Build history of the part. All positions in model axes, mm. Face numbers are marked on the shaded views. A direction names the side the tool comes from. Give positions to 0.01 mm unless a question says otherwise; leave off trailing zeros. Loops run counter-clockwise (first coordinate to the right, second up) from the corner with the lowest first, then second, coordinate; pieces in that order, holes last. Notation, with made-up numbers: (51, 8.5) -> (109, 8.5) arc R13 ccw to (109, 13.5) -> close; hole circle Ø6 at (51, 63.5). An arc over 180 degrees is marked (long way). Answer in a Markdown table with one row per item. Add a question column.
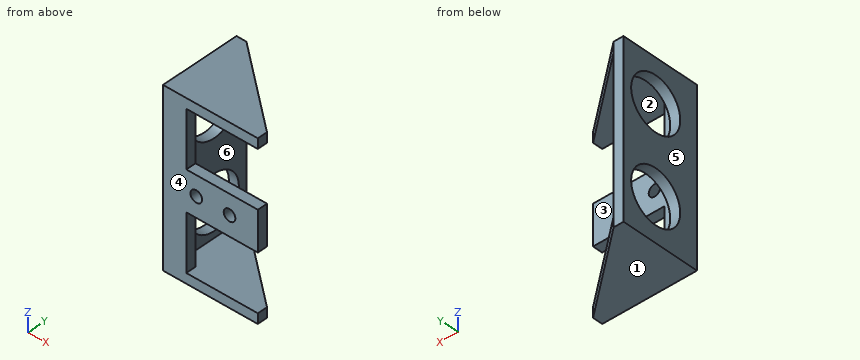
from build123d import *

# Parameters (mm, degrees)
CROQUIS1_W              = 52
CROQUIS1_H              = 21
CROQUIS1_R              = 8.025
SALIENTE_EXTRUIR1_DEPTH = 3
CROQUIS2_W              = 3
CROQUIS2_H              = 21
SALIENTE_EXTRUIR2_DEPTH = 28.5
CORTAR_EXTRUIR1_DEPTH   = 61.815294129
CROQUIS4_R              = 1.75
CORTAR_EXTRUIR2_DEPTH   = 53.671149598
CROQUIS5_W              = 21.5
CROQUIS5_H              = 17
CORTAR_EXTRUIR3_DEPTH   = 53.671149598


with BuildPart() as part:
    # Croquis1 → Saliente-Extruir1 (new body)
    with BuildSketch(Plane(origin=(0, 0, 0), x_dir=(0, 0, -1), z_dir=(1, 0, 0))):
        with Locations((13, 0)):
            Rectangle(CROQUIS1_W, CROQUIS1_H)
        Circle(CROQUIS1_R, mode=Mode.SUBTRACT)
        with Locations((26, 0)):
            Circle(CROQUIS1_R, mode=Mode.SUBTRACT)
    extrude(amount=SALIENTE_EXTRUIR1_DEPTH)

    # Croquis2 → Saliente-Extruir2 (add)
    with BuildSketch(Plane.ZY):
        Polygon((-36, -10.5), (-39, -10.5), (-39, -13.5), (13, -13.5), (13, -10.5), (10, -10.5), align=None)
        with Locations((11.5, 0)):
            Rectangle(CROQUIS2_W, CROQUIS2_H)
        with Locations((-37.5, 0)):
            Rectangle(CROQUIS2_W, CROQUIS2_H)
    extrude(amount=-SALIENTE_EXTRUIR2_DEPTH)

    # Croquis3 → Cortar-Extruir1 (cut, through all)
    with BuildSketch(Plane.XY.offset(13)):
        Polygon((3, 10.5), (28.5, -10.5), (28.5, 10.5), align=None)
    extrude(amount=-CORTAR_EXTRUIR1_DEPTH, mode=Mode.SUBTRACT)

    # Croquis4 → Cortar-Extruir2 (cut, through all)
    with BuildSketch(Plane(origin=(0, -10.5, 0), x_dir=(1, 0, 0), z_dir=(0, 1, 0))):
        with Locations(Location((10, 13, 0), (0, 0, 270))):
            Circle(CROQUIS4_R)
        with Locations(Location((20, 13, 0), (0, 0, 270))):
            Circle(CROQUIS4_R)
    extrude(amount=-CORTAR_EXTRUIR2_DEPTH, mode=Mode.SUBTRACT)

    # Croquis5 → Cortar-Extruir3 (cut, through all)
    with BuildSketch(Plane(origin=(0, -10.5, 0), x_dir=(1, 0, 0), z_dir=(0, 1, 0))):
        with Locations((17.75, 27.5)):
            Rectangle(CROQUIS5_W, CROQUIS5_H)
        with Locations((17.75, -1.5)):
            Rectangle(CROQUIS5_W, CROQUIS5_H)
    extrude(amount=-CORTAR_EXTRUIR3_DEPTH, mode=Mode.SUBTRACT)


solid = part.part
(1) Two-plate mould, pull along Z, no slides. Class the marked faces 1, 2, 3 and 4: released by +Z, released by -Z, zero draft, split by the parting line, or undercut.
(2) Saw through at B-B, the plane z = -26. List the corners of the cut face in (x, y) (3 decimals).
(3) 3-axis set-ups, long thin cutter, end or side, ignore diameter. For the marked faces 5 and 6: which of +Z, -Z, +X, -X, +Y, -Y reach the whole face in a straight line?
(4) Flat gauge pins, fed straight in: pin 1 Ø12 at (x, y) = (20, 4.5) entering from -Z; pin 2 Ø5 at (y, z) = (-6.5, 6) entering from +X; pin 3 Ø3.5 at (y, z) = (-12, -30) entering from +X; pin 4 Ø4 at (x, z) = (10, -13) entering from +Y. Where does each tip first touch, or does it go through?
(5) Saw through at A-A, the plane y = 0. List the corners of the cut face in (x, z) (3 decimals), then the cut area to 3 significant figures.
(6) Saw through at C-C, the plane x = 20. List the corners of the cut face in (y, z), then the cut area to 3 significant figures.
(7) Wall check: line 1 along Z through (x, y) = (22, -12.25); line 2 along Z through (x, y) = (14, -10); line 3 along X through (y, z) = (-12.5, -13). Give the ranges that are in metal, low to high. Write a range as from..to.
(8) Saw through at D-D, the plane z = -13. List the corners of the cut face in (x, y).
Worked answers:
| question | item | result |
|---|---|---|
| 1 | face 1 | released by -Z |
| 1 | face 2 | undercut |
| 1 | face 3 | undercut |
| 1 | face 4 | zero draft |
| 2 | outline | (0, -13.5) -> (7, -13.5) -> (7, -10.5) -> (3, -10.5) -> (3, -8.025) -> (0, -8.025) -> close; (0, 8.025) -> (3, 8.025) -> (3, 10.5) -> (0, 10.5) -> close |
| 3 | face 5 | +Z, -Z, -X, +Y, -Y |
| 3 | face 6 | +X, +Y |
| 4 | pin 1 | through |
| 4 | pin 2 | x = 3 |
| 4 | pin 3 | x = 7 |
| 4 | pin 4 | y = -10.5 |
| 5 | outline | (0, -39) -> (15.75, -39) -> (15.75, -36) -> (3, -36) -> (3, -34.025) -> (0, -34.025) -> close; (0, -17.975) -> (3, -17.975) -> (3, -8.025) -> (0, -8.025) -> close; (0, 8.025) -> (3, 8.025) -> (3, 10) -> (15.75, 10) -> (15.75, 13) -> (0, 13) -> close |
| 5 | area | 136 mm^2 |
| 6 | outline | (-13.5, -39) -> (-3.5, -39) -> (-3.5, -36) -> (-13.5, -36) -> close; (-13.5, -19) -> (-10.5, -19) -> (-10.5, -14.75) -> (-13.5, -14.75) -> close; (-13.5, -11.25) -> (-10.5, -11.25) -> (-10.5, -7) -> (-13.5, -7) -> close; (-13.5, 10) -> (-3.5, 10) -> (-3.5, 13) -> (-13.5, 13) -> close |
| 6 | area | 85.5 mm^2 |
| 7 | line 1 | -39..-36, -19..-7, 10..13 |
| 7 | line 2 | -39..-36, 10..13 |
| 7 | line 3 | 0..8.25, 11.75..18.25, 21.75..28.5 |
| 8 | outline | (0, -13.5) -> (8.25, -13.5) -> (8.25, -10.5) -> (3, -10.5) -> (3, 10.5) -> (0, 10.5) -> close; (11.75, -13.5) -> (18.25, -13.5) -> (18.25, -10.5) -> (11.75, -10.5) -> close; (21.75, -13.5) -> (28.5, -13.5) -> (28.5, -10.5) -> (21.75, -10.5) -> close |
